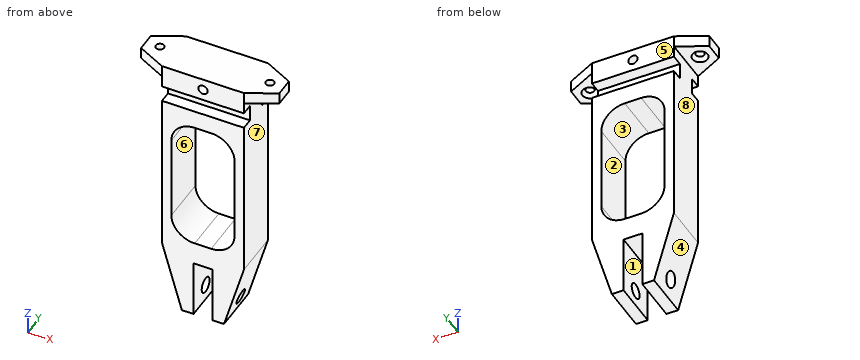
```python
from build123d import *

# Parameters (mm, degrees)
CROQUIS1_R                 = 3.25
SALIENTE_EXTRUIR1_DEPTH    = 35
CORTAR_EXTRUIR1_REACH      = 125.844
CROQUIS2_W                 = 8
CROQUIS2_H                 = 25
CROQUIS4_W                 = 27
CROQUIS4_H                 = 57
CORTAR_EXTRUIR2_DEPTH      = 124.844297406
CORTAR_EXTRUIR3_REACH      = 125.844
CROQUIS9_R                 = 1.75
SALIENTE_EXTRUIR3_DEPTH    = 5
CHAFL_N1_SIZE              = 1.5
CHAFL_N1_OF_SIMETR_A3_SIZE = 1.5
ENGANCHE_REACH             = 129.755
CROQUIS7_R                 = 2
REDONDEO1_R                = 10


with BuildPart() as part:
    # Croquis1 → Saliente-Extruir1 (new body)
    with BuildSketch(Plane(origin=(0, 0, 0), x_dir=(0, 0, -1), z_dir=(1, 0, 0))):
        Polygon((0, 10), (0, -10), (10, -10), (10, -5), (17.1, -5), (17.1, -10), (117.1, -10), (117.1, 10), (17.1, 10), (17.1, 5), (10, 5), (10, 10), align=None)
        with Locations((110.1, 0)):
            Circle(CROQUIS1_R, mode=Mode.SUBTRACT)
    extrude(amount=SALIENTE_EXTRUIR1_DEPTH)

    # Croquis2 → Cortar-Extruir1 (cut, up to next)
    with BuildSketch(Plane(origin=(0, 10, 0), x_dir=(1, 0, 0), z_dir=(0, 1, 0)), mode=Mode.PRIVATE) as cortar_extruir1_sk1:
        with Locations((17.5, 104.6)):
            Rectangle(CROQUIS2_W, CROQUIS2_H)
    cortar_extruir1_tool1 = extrude(cortar_extruir1_sk1.sketch, amount=-CORTAR_EXTRUIR1_REACH, mode=Mode.PRIVATE) & part.part
    add(cortar_extruir1_tool1.solids().sort_by_distance((17.5, 10, -104.6))[0], mode=Mode.SUBTRACT)

    # Croquis4 → Cortar-Extruir2 (cut, through all)
    with BuildSketch(Plane(origin=(0, 10, 0), x_dir=(1, 0, 0), z_dir=(0, 1, 0))):
        with Locations((17.5, 53.6)):
            Rectangle(CROQUIS4_W, CROQUIS4_H)
    extrude(amount=-CORTAR_EXTRUIR2_DEPTH, mode=Mode.SUBTRACT)

    # Croquis5 → Cortar-Extruir3 (cut, up to next)
    with BuildSketch(Plane(origin=(0, 10, 0), x_dir=(1, 0, 0), z_dir=(0, 1, 0)), mode=Mode.PRIVATE) as cortar_extruir3_sk1:
        Polygon((8.5, 117.1), (0, 87.1), (0, 117.1), align=None)
    cortar_extruir3_tool1 = extrude(cortar_extruir3_sk1.sketch, amount=-CORTAR_EXTRUIR3_REACH, mode=Mode.PRIVATE) & part.part
    cortar_extruir3 = cortar_extruir3_tool1.solids().sort_by_distance((2.833333, 10, -107.1))[0]
    add(cortar_extruir3, mode=Mode.SUBTRACT)

    # Simetría1: Cortar-Extruir3 across plane
    add(cortar_extruir3.mirror(Plane(origin=(17.5, 0, 0), x_dir=(0, 0, 1), z_dir=(1, 0, 0))), mode=Mode.SUBTRACT)

    # Croquis9 → Saliente-Extruir3 (add)
    with BuildSketch(Plane.XY):
        Polygon((0, 10), (-12, 4), (-12, -4), (0, -10), align=None)
        with Locations((-6, 0)):
            Circle(CROQUIS9_R, mode=Mode.SUBTRACT)
    saliente_extruir3 = extrude(amount=-SALIENTE_EXTRUIR3_DEPTH)

    # Chaflán1
    chafl_n1_edges = [part.edges().sort_by_distance(p)[0] for p in [
        (-7.75, 0, -5),
    ]]
    chamfer(chafl_n1_edges, length=CHAFL_N1_SIZE)

    # Simetría3: Saliente-Extruir3 across plane
    add(saliente_extruir3.mirror(Plane(origin=(17.5, 0, 0), x_dir=(0, 0, 1), z_dir=(1, 0, 0))))

    # Chaflán1 of Simetría3
    chafl_n1_of_simetr_a3_edges = [part.edges().sort_by_distance(p)[0] for p in [
        (42.75, 0, -5),
    ]]
    chamfer(chafl_n1_of_simetr_a3_edges, length=CHAFL_N1_OF_SIMETR_A3_SIZE)

    # Croquis7 → Enganche (cut, up to next)
    with BuildSketch(Plane(origin=(0, 10, 0), x_dir=(1, 0, 0), z_dir=(0, 1, 0)), mode=Mode.PRIVATE) as enganche_sk1:
        with Locations(Location((17.5, 5, 0), (0, 0, 270))):
            Circle(CROQUIS7_R)
    enganche_tool1 = extrude(enganche_sk1.sketch, amount=-ENGANCHE_REACH, mode=Mode.PRIVATE) & part.part
    add(enganche_tool1.solids().sort_by_distance((17.5, 10, -5))[0], mode=Mode.SUBTRACT)

    # Redondeo1
    redondeo1_edges = [part.edges().sort_by_distance(p)[0] for p in [
        (31, 0, -82.1),
        (31, 0, -25.1),
        (4, 0, -25.1),
        (4, 0, -82.1),
    ]]
    fillet(redondeo1_edges, radius=REDONDEO1_R)


solid = part.part
```
Could you check a few things on this model? Use its own coordinates, in mm. Face numbers are marked on the shaded views. A direction names the side the tool comes from. Round coordinates to 2 decimals unless told otherwise and drop trailing zeros. Loops run counter-clockwise (first coordinate to the right, second up) from the corner with the lowest first, then second, coordinate; pieces in that order, holes last. Notation, with made-up numbers: (54, -36.5) - (80, -36.5) arc R8 cw to (80, -29.5) - close; hole circle Ø4 at (84, 70.25). An arc over 180 degrees is marked (long way). Answer in a Markdown table with one row per item. Add a question column.
(1) If we section it at A-A (z = -44.5): Please give me the cut outline in (x, y), plus the area to 3 significant figures.
(2) If we section it at B-B (x = -6): Please give me the cut outline in (y, z).
(3) If we section it at D-D (z = -110.1): Please give me the cut outline in (x, y), plus the area to 3 significant figures.
(4) If we mould it in two halves opening along Z, with no side actions, what happens to the marked faces 1, 2, 3 and 4? For each: pulls with the +Z half, pulls with the -Z half, needs draft (parallel to the pull), parting line crosses it, or undercut.
(5) I need wall thicknesses on line 1 along Z through (x, y) = (24.5, -2); line 2 along Z through (x, y) = (25, 2.25); line 3 along Y through (x, z) = (10.75, -110.1). Which ranges of each line are inside material? Lowest first, please.
(6) For the marked faces 5, 6, 7 and 8, which set-ups out of +Z, -Z, +X, -X, +Y, -Y let a thin tool reach every point of the face, with its end or its side?
(7) If we section it at C-C (x = 24): Please give me the cut outline in (y, z), plus the area to 3 significant figures.
(8) I'm going to push flat-ended pins straight in: pin 1 (9.5 mm diameter, centred on x = -5.5, y = 4.5, fed in from -Z); pin 2 (10 mm diameter, centred on y = 3, z = -42, fed in from -X); pin 3 (6 mm diameter, centred on y = -2.5, z = -48, fed in from +X); pin 4 (4.5 mm diameter, centred on x = 17.5, z = -5, fed in from -Y). Where does each tip first touch, or does it pass through?
Model answer:
| question | item | result |
|---|---|---|
| 1 | outline | (0, -10) - (4, -10) - (4, 10) - (0, 10) - close; (31, -10) - (35, -10) - (35, 10) - (31, 10) - close |
| 1 | area | 160 mm² |
| 2 | outline | (-7, -5) - (-3.25, -5) - (-1.75, -3.5) - (-1.75, 0) - (-7, 0) - close; (1.75, -3.5) - (3.25, -5) - (7, -5) - (7, 0) - (1.75, 0) - close |
| 3 | outline | (6.52, -10) - (13.5, -10) - (13.5, -3.25) - (6.52, -3.25) - close; (6.52, 3.25) - (13.5, 3.25) - (13.5, 10) - (6.52, 10) - close; (21.5, -10) - (28.48, -10) - (28.48, -3.25) - (21.5, -3.25) - close; (21.5, 3.25) - (28.48, 3.25) - (28.48, 10) - (21.5, 10) - close |
| 3 | area | 189 mm² |
| 4 | face 1 | needs draft |
| 4 | face 2 | undercut |
| 4 | face 3 | undercut |
| 4 | face 4 | pulls with the -Z half |
| 5 | line 1 | z = -117.1 to -112.66, -107.54 to -81.47, -25.73 to 0 |
| 5 | line 2 | z = -117.1 to -112.45, -107.75 to -81.27, -25.93 to 0 |
| 5 | line 3 | y = -10 to -3.25, 3.25 to 10 |
| 6 | face 5 | +Z, -Z, +X, -X, +Y |
| 6 | face 6 | +Y, -Y |
| 6 | face 7 | -Z, +X, +Y, -Y |
| 6 | face 8 | -Z, -X, +Y, -Y |
| 7 | outline | (-10, -117.1) - (10, -117.1) - (10, -81.64) - (-10, -81.64) - close; (-10, -25.56) - (10, -25.56) - (10, -17.1) - (5, -17.1) - (5, -10) - (10, -10) - (10, 0) - (-10, 0) - (-10, -10) - (-5, -10) - (-5, -17.1) - (-10, -17.1) - close; hole circle Ø6.5 at (0, -110.1) |
| 7 | area | 1,120 mm² |
| 8 | pin 1 | stops at z = -5 |
| 8 | pin 2 | stops at x = 0 |
| 8 | pin 3 | stops at x = 35 |
| 8 | pin 4 | stops at y = -10 |
